Autodesk Inventor part; units mm, degrees
ref_plane "YZ Plane" through (0, 0, 0) normal (1, 0, 0) x (0, 1, 0)
ref_plane "XZ Plane" through (0, 0, 0) normal (0, 1, 0) x (-1, 0, 0)
ref_plane "XY Plane" through (0, 0, 0) normal (0, 0, 1) x (1, 0, 0)
sketch "Sketch1" plane through (0, 0, 0) normal (0, 1, 0) x (-1, 0, 0)
  line L0 (38, 79) -> (-38, 79)
  line L1 (-38, 79) -> (-38, -79)
  line L2 (-38, -79) -> (38, -79)
  line L3 (38, -79) -> (38, 79)
  line L4 (0, 0) -> (38, 0) construction
  line L5 (0, 0) -> (0, -79) construction
  dimension "d0" = 158
  dimension "d1" = 76
extrude "Extrusion1" add sketch "Sketch1" along normal blind 9.525
sketch "Sketch2" plane through (0, 0, 0) normal (0, -1, 0) x (1, 0, 0)
  line L0 (-38, 79) -> (38, 79) construction
  line L1 (-38, -79) -> (-38, 79) construction
  line L2 (38, -79) -> (-38, -79) construction
  line L3 (38, 79) -> (38, -79) construction
  line L4 (-6, -25.4) -> (-6, 25.4) construction
  line L5 (-38, 0) -> (38, 0) construction
  line L6 (25.75, -25.4) -> (25.75, 25.4) construction
  point P0 (0, 0)
  point P1 (-6, 0)
  point P2 (25.75, 0)
  dimension "d4" = 50.8
  dimension "d5" = 50.8
  dimension "d6" = 31.75
  dimension "d16" = 32
hole "Hole1" at (-6, 0, 25.4) at (25.75, 0, 25.4) at (25.75, 0, -25.4) at (-6, 0, -25.4) direction (0, 1, 0) diameter 6.756 end through all counterbore diameter 11.113 counterbore depth 6.35
sketch "Sketch3" plane through (0, 9.525, 0) normal (0, 1, 0) x (1, 0, 0)
  line L0 (38, -79) -> (38, 79) construction
  line L1 (38, 79) -> (-38, 79) construction
  line L2 (-38, 79) -> (-38, -79) construction
  line L3 (-38, -79) -> (38, -79) construction
  line L4 (-31.65, 79) -> (-31.65, -79) construction
  point P0 (0, 0)
  point P1 (-31.65, 47.4)
  point P2 (-31.65, 15.8)
  point P3 (-31.65, -47.4)
  point P4 (-31.65, -15.8)
  dimension "d17" = 6.35
  dimension "d19" = 31.6
  dimension "d20" = 31.6
  dimension "d21" = 31.6
  dimension "d22" = 31.6
  dimension "d23" = 31.6
hole "Hole2" at (-31.65, 9.525, -47.4) at (-31.65, 9.525, -15.8) at (-31.65, 9.525, 47.4) at (-31.65, 9.525, 15.8) direction (0, -1, 0) diameter 6.756 end through all counterbore diameter 11.113 counterbore depth 6.35
properties part number "base_part"
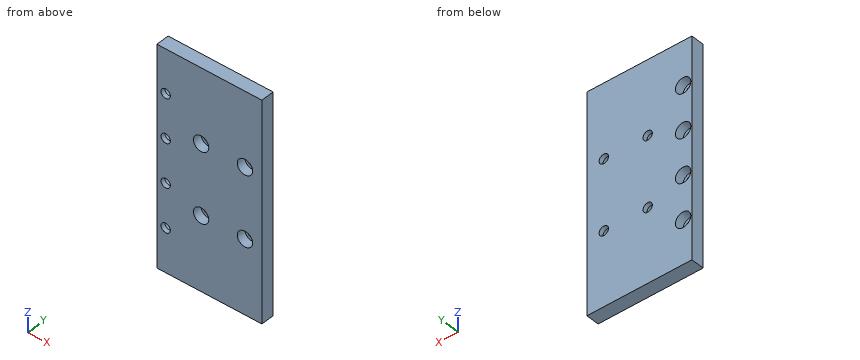
CAD build for the part. Positions are in the model's coordinates, mm. Round coordinates to 2 decimals unless told otherwise and drop trailing zeros. Order: outer loops, then holes, each group sorted by start corner. A loop starts at its lowest first (then second) coordinate and runs counter-clockwise, first axis right, second up. Notation, with made-up numbers: (84, 9.25) - (112, 9.25) arc R22 cw to (112, 45.25) - close; hole circle Ø6 at (-8.75, 40). An arc over 180 degrees is marked (long way). Answer as CSV lines item,"result". Start each with the question number.
1. Drill centre lines: L1, parallel to Z at x = 25.75, y = 4; L2, parallel to Z at x = -31.65, y = 6; L3, parallel to X at y = 4.5, z = -15.8. Where is each one in solid material? Low to high. Write a range as [from, to].
2. Pin check, flat tips, straight feed: pin 1 (10 mm diameter, centred on x = -31.65, z = -47.4, fed in from +Y) (3 decimals); pin 2 (3.5 mm diameter, centred on x = -8.5, z = 26, fed in from -Y). Stop position of each tip, or through.
3. Saw through at B-B, the plane x = -6. Count the separate pieces of the cut face and the enclosed holes in it, and give its area (3 significant figures).
4. Saw through at A-A, the plane z = -47.4. Write the cut outline in (x, y) (1 decimal), and give its area (3 significant figures).
Model answer:
1,L1,"z = [-79, -30.96], [-19.84, 19.84], [30.96, 79]"
1,L2,"z = [-79, -52.96], [-41.84, -21.36], [-10.24, 10.24], [21.36, 41.84], [52.96, 79]"
1,L3,"x = [-38, -37.21], [-26.09, 38]"
2,pin 1,"stops at y = 3.175"
2,pin 2,"stops at y = 6.35"
3,separate pieces,"3"
3,enclosed holes,"0"
3,area,"1,320 mm²"
4,outline,"(-38, 0) - (-35, 0) - (-35, 3.2) - (-37.2, 3.2) - (-37.2, 9.5) - (-38, 9.5) - close; (-28.3, 0) - (38, 0) - (38, 9.5) - (-26.1, 9.5) - (-26.1, 3.2) - (-28.3, 3.2) - close"
4,area,"632 mm²"
